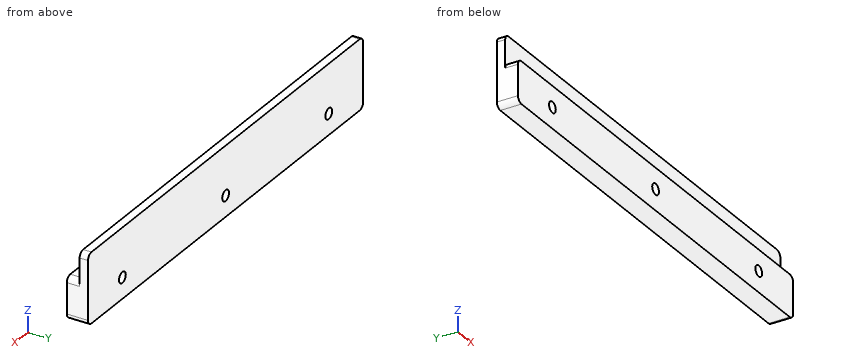
from build123d import *

# Parameters (mm, degrees)
EXTRUDE_1_DEPTH     = 160
CUT_EXTRUDE_1_REACH = 164.12
SKETCH_2_R          = 1.95
FILLET_1_R          = 2


with BuildPart() as part:
    # 草图1 → 凸台-拉伸1 (new body)
    with BuildSketch(Plane(origin=(0, 0, 0), x_dir=(0, 0, -1), z_dir=(1, 0, 0))):
        Polygon((0, 0), (0, 7.6), (-25, 7.6), (-25, 4.6), (-15, 4.6), (-15, 0), align=None)
    extrude(amount=EXTRUDE_1_DEPTH)

    # 草图2 → 切除-拉伸1 (cut, up to next)
    with BuildSketch(Plane.XZ, mode=Mode.PRIVATE) as cut_extrude_1_sk1:
        with Locations(Location((20, 7.5, 0), (0, 0, 270))):
            Circle(SKETCH_2_R)
    cut_extrude_1_tool1 = extrude(cut_extrude_1_sk1.sketch, amount=-CUT_EXTRUDE_1_REACH, mode=Mode.PRIVATE) & part.part
    # 草图2 → 切除-拉伸1 (cut, up to next)
    with BuildSketch(Plane.XZ, mode=Mode.PRIVATE) as cut_extrude_1_sk2:
        with Locations(Location((140, 7.5, 0), (0, 0, 270))):
            Circle(SKETCH_2_R)
    cut_extrude_1_tool2 = extrude(cut_extrude_1_sk2.sketch, amount=-CUT_EXTRUDE_1_REACH, mode=Mode.PRIVATE) & part.part
    # 草图2 → 切除-拉伸1 (cut, up to next)
    with BuildSketch(Plane.XZ, mode=Mode.PRIVATE) as cut_extrude_1_sk3:
        with Locations(Location((80, 7.5, 0), (0, 0, 270))):
            Circle(SKETCH_2_R)
    cut_extrude_1_tool3 = extrude(cut_extrude_1_sk3.sketch, amount=-CUT_EXTRUDE_1_REACH, mode=Mode.PRIVATE) & part.part
    add(cut_extrude_1_tool1.solids().sort_by_distance((20, 0, 7.5))[0], mode=Mode.SUBTRACT)
    add(cut_extrude_1_tool2.solids().sort_by_distance((140, 0, 7.5))[0], mode=Mode.SUBTRACT)
    add(cut_extrude_1_tool3.solids().sort_by_distance((80, 0, 7.5))[0], mode=Mode.SUBTRACT)

    # 圆角1
    fillet_1_edges = [part.edges().sort_by_distance(p)[0] for p in [
        (160, 6.1, 25),
        (160, 2.3, 15),
        (0, 2.3, 15),
        (0, 6.1, 25),
        (0, 3.8, 0),
        (160, 3.8, 0),
    ]]
    fillet(fillet_1_edges, radius=FILLET_1_R)


solid = part.part
Can you work these out from the model? Positions are in its coordinate system, mm. Give positions to 0.01 mm unless a question says otherwise; leave off trailing zeros. Order: outer loops, then holes, each group sorted by start corner. A loop starts at its lowest first (then second) coordinate and runs counter-clockwise, first axis right, second up. Notation, with made-up numbers: M 82.25,19.25 L 95.25,19.25 A11 cw 95.25,29.25 Z; hole C 13.5,71 d11. An arc over 180 degrees is marked long. One line per item, written item: value.
Item 1: Please list where these lines run through material, in increasing order: line 1 (X direction, y = 4.75, z = 7.5); line 2 (Z direction, x = 140, y = 5); line 3 (Y direction, x = 20, z = 15.5).
Verdict:
line 1: 0 to 18.05, 21.95 to 78.05, 81.95 to 138.05, 141.95 to 160
line 2: 0 to 5.55, 9.45 to 25
line 3: 4.6 to 7.6
Item 2: If we section it at D-D on z = 18.5: Write out the boundary of the cut face in (x, y), and give its area (3 significant figures).
Verdict:
outline: M 0,4.6 L 160,4.6 L 160,7.6 L 0,7.6 Z
area: 480 mm2
Item 3: If we section it at A-A on x = 20: Write out the boundary of the cut face in (y, z), and give its area (3 significant figures).
Verdict:
outline: M 0,0 L 7.6,0 L 7.6,5.55 L 0,5.55 Z; M 0,9.45 L 7.6,9.45 L 7.6,25 L 4.6,25 L 4.6,15 L 0,15 Z
area: 114 mm2
Item 4: If we section it at B-B on z = 7.5: Write out the boundary of the cut face in (x, y).
Verdict:
outline: M 0,0 L 18.05,0 L 18.05,7.6 L 0,7.6 Z; M 21.95,0 L 78.05,0 L 78.05,7.6 L 21.95,7.6 Z; M 81.95,0 L 138.05,0 L 138.05,7.6 L 81.95,7.6 Z; M 141.95,0 L 160,0 L 160,7.6 L 141.95,7.6 Z
Item 5: If we section it at C-C on y = 1.75: Write out the boundary of the cut face in (x, z), and give its area (3 significant figures).
Verdict:
outline: M 0,2 A2 ccw 2,0 L 158,0 A2 ccw 160,2 L 160,13 A2 ccw 158,15 L 2,15 A2 ccw 0,13 Z; hole C 20,7.5 d3.9; hole C 80,7.5 d3.9; hole C 140,7.5 d3.9
area: 2,360 mm2
Item 6: For pin 1 (2.5 mm diameter, centred on x = 57.5, y = 3.5, fed in from +Z); pin 2 (1.5 mm diameter, centred on x = 83.5, z = 22, fed in from -Y), each with a flat end and sliding along its axis, tell me the tip position at first contact or that it passes through.
Verdict:
pin 1: z = 25
pin 2: y = 4.6
